Read the model definition and answer for the solid it produces. Units are mm, in the model's axes. A direction names the side the tool comes from. Round coordinates to 2 decimals unless told otherwise and drop trailing zeros. Write each loop counter-clockwise with the first axis right and the second up, starting at its lowest first coordinate (ties: lowest second). Pieces come first, ordered by that corner, then holes.
from build123d import *

# Parameters (mm, degrees)
F0_R     = 10.115
F0_R_2   = 4.71
F1_DEPTH = 25.4
F0_R_3   = 2.25
F2_DEPTH = 19.05
F3_DEPTH = 3.034123


with BuildPart() as f1:
    # F0 (on Front) → F1 (new body)
    with BuildSketch(Plane.XZ):
        Circle(F0_R)
        Circle(F0_R_2, mode=Mode.SUBTRACT)
    extrude(amount=F1_DEPTH)

    # F0 (on Front) → F2 (join)
    with BuildSketch(Plane.XZ):
        Circle(F0_R_2)
        Circle(F0_R_3, mode=Mode.SUBTRACT)
    extrude(amount=F2_DEPTH)

    # F0 (on Front) → F3 (cut)
    with BuildSketch(Plane.XZ):
        Circle(F0_R_2)
        Circle(F0_R_3, mode=Mode.SUBTRACT)
    extrude(amount=F3_DEPTH, mode=Mode.SUBTRACT)


solid = f1.part
Q1. Section A-A (x = 0) is taken. Determine the outline of the cut face in (y, z) (3 decimals), then the cut area to 3 significant figures.
Verdict:
outline: (-25.4, -10.115) - (0, -10.115) - (0, -4.71) - (-3.034, -4.71) - (-3.034, -2.25) - (-19.05, -2.25) - (-19.05, -4.71) - (-25.4, -4.71) - close; (-25.4, 4.71) - (-19.05, 4.71) - (-19.05, 2.25) - (-3.034, 2.25) - (-3.034, 4.71) - (0, 4.71) - (0, 10.115) - (-25.4, 10.115) - close
area: 353 mm2
Q2. Flat-ended cylindrical pins translate along their axes: pin 1 Ø10 at (y, z) = (-10, 3) entering from -X (3 decimals); pin 2 Ø2 at (x, y) = (-8, -6) entering from -Z; pin 3 Ø1.5 at (y, z) = (-9, 2) entering from +X; pin 4 Ø1 at (x, y) = (6.5, -11) entering from -Z. Find the tip coordinate at first contact, or state that the pin passes through.
Verdict:
pin 1: stops at x = -10.115
pin 2: stops at z = -7.3
pin 3: stops at x = 10.04
pin 4: stops at z = -8.14
Q3. Section C-C (y = -10.5) is taken. Determine the outline of the cut face in (x, z) (3 decimals).
Verdict:
outline: circle Ø20.23 at (0, 0); hole circle Ø4.5 at (0, 0)
Q4. Section B-B (z = 0) is taken. Determine the outline of the cut face in (x, y) (3 decimals).
Verdict:
outline: (-10.115, -25.4) - (-4.71, -25.4) - (-4.71, -19.05) - (-2.25, -19.05) - (-2.25, -3.034) - (-4.71, -3.034) - (-4.71, 0) - (-10.115, 0) - close; (2.25, -19.05) - (4.71, -19.05) - (4.71, -25.4) - (10.115, -25.4) - (10.115, 0) - (4.71, 0) - (4.71, -3.034) - (2.25, -3.034) - close
Q5. Determine the mould class of faces 1 (the flat face through (2.1, 0, -4.4)), 2 (the flat face through (1, -3.034, 2.2)), 3 (the cylindrical face through (-1.32, -12.52, 10.03)) for opening direction X: pulls with the +X half, pulls with the -X half, needs draft (parallel to the pull), parting line crosses it, or undercut.
Verdict:
face 1: needs draft
face 2: undercut
face 3: parting line crosses it
Q6. Which of the six approach directions +Z, -Z, +X, -X, +Y, -Y give full straight-line access (tool end or side, diameter ignored) to faces 4 (the flat face through (4.4, -25.4, -2.1)), 5 (the cylindrical face through (-1.02, -1.5, -4.6)), 6 (the flat face through (1, -19.05, 2.2))?
Verdict:
face 4: +Z, -Z, +X, -X, -Y
face 5: +Y
face 6: -Y
Q7. Straight lines are drawn through the part: probe 1 along Z at (x, y) = (0, -23.75) (3 decimals); probe 2 along Z at (x, y) = (0, -14.75) (3 decimals); probe 3 along X at (y, z) = (-19.75, -3.25). For each, find the intervals that lie inside material, in ascending order.
Verdict:
probe 1: z = -10.115 to -4.71, 4.71 to 10.115
probe 2: z = -10.115 to -2.25, 2.25 to 10.115
probe 3: x = -9.58 to -3.41, 3.41 to 9.58
Q8. Section D-D (x = 4) is taken. Determine the outline of the cut face in (y, z), then the cut area to 3 significant figures.
Verdict:
outline: (-25.4, -9.29) - (0, -9.29) - (0, -2.49) - (-3.03, -2.49) - (-3.03, 2.49) - (0, 2.49) - (0, 9.29) - (-25.4, 9.29) - (-25.4, 2.49) - (-19.05, 2.49) - (-19.05, -2.49) - (-25.4, -2.49) - close
area: 425 mm2
